Part model, mm, in its own coordinate system. Face numbers are marked on the shaded views. A direction names the side the tool comes from. Give positions to 0.01 mm unless a question says otherwise; leave off trailing zeros. Write each loop counter-clockwise with the first axis right and the second up, starting at its lowest first coordinate (ties: lowest second). Pieces come first, ordered by that corner, then holes.
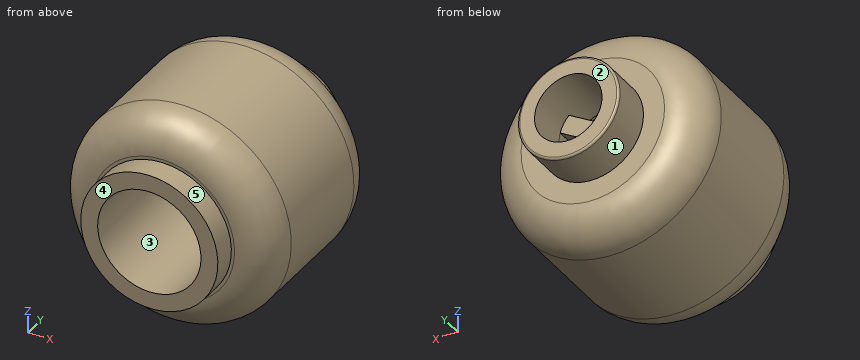
```python
from build123d import *

# Parameters (mm, degrees)
FILLET1_R          = 1.7
SKETCH2_R          = 1.6
CUT_EXTRUDE1_DEPTH = 2
CUT_EXTRUDE2_DEPTH = 13.0074977
SKETCH4_R          = 2.45
CUT_EXTRUDE3_DEPTH = 8.5
FILLET2_R          = 0.1


with BuildPart() as part:
    # Sketch1 → Revolve1 (revolve)
    with BuildSketch(Plane.XY, mode=Mode.PRIVATE) as revolve1_sk:
        Polygon((0, 11.6), (2.4, 11.6), (2.4, 9.6), (5.1, 9.6), (5.1, 1.1), (3.25, 1.1), (3.25, 0), (0, 0), align=None)
    revolve(revolve1_sk.sketch.rotate(Axis((0, 161.315789474, 0), (0, -1, 0)), 90), axis=Axis((0, 161.315789474, 0), (0, -1, 0)))

    # Fillet1
    fillet1_edges = [part.edges().sort_by_distance(p)[0] for p in [
        (0, 1.1, -5.1),
        (0, 9.6, -5.1),
    ]]
    fillet(fillet1_edges, radius=FILLET1_R)

    # Sketch2 → Cut-Extrude1 (cut)
    with BuildSketch(Plane(origin=(0, 11.6, 0), x_dir=(1, 0, 0), z_dir=(0, 1, 0))):
        with Locations(Location((0, 0, 0), (0, 0, 270))):
            Circle(SKETCH2_R)
    extrude(amount=-CUT_EXTRUDE1_DEPTH, mode=Mode.SUBTRACT)

    # Sketch3 → Cut-Extrude2 (cut, through all)
    with BuildSketch(Plane(origin=(0, 9.6, 0), x_dir=(1, 0, 0), z_dir=(0, 1, 0))):
        with BuildLine():
            Line((-0.42, 0.242487113), (-0.42, 1.543891188))
            ThreePointArc((-0.42, 1.543891188), (-1.385640646, 0.8), (-1.547048989, -0.408214924))
            Line((-1.547048989, -0.408214924), (-0.42, 0.242487113))
        make_face()
        with BuildLine():
            ThreePointArc((1.6, 0), (1.271219887, 0.971596624), (0.42, 1.543891188))
            Line((0.42, 1.543891188), (0.42, 0.242487113))
            Line((0.42, 0.242487113), (1.547048989, -0.408214924))
            ThreePointArc((1.547048989, -0.408214924), (1.586707028, -0.205817415), (1.6, 0))
        make_face()
        with BuildLine():
            Line((0, -0.484974226), (-1.127048989, -1.135676264))
            ThreePointArc((-1.127048989, -1.135676264), (0, -1.6), (1.127048989, -1.135676264))
            Line((1.127048989, -1.135676264), (0, -0.484974226))
        make_face()
    extrude(amount=-CUT_EXTRUDE2_DEPTH, mode=Mode.SUBTRACT)

    # Sketch4 → Cut-Extrude3 (cut)
    with BuildSketch(Plane.XZ):
        with Locations(Location((0, 0, 0), (0, 0, 270))):
            Circle(SKETCH4_R)
    extrude(amount=-CUT_EXTRUDE3_DEPTH, mode=Mode.SUBTRACT)

    # Fillet2
    fillet2_edges = [part.edges().sort_by_distance(p)[0] for p in [
        (0, 11.6, -2.4),
    ]]
    fillet(fillet2_edges, radius=FILLET2_R)


solid = part.part
```
1) Saw through at B-B, the plane x = 0.75. Count the separate pieces of the cut face and the enclosed holes in it, then the cut area to 3 significant figures.
Answers follow:
separate pieces: 3
enclosed holes: 0
area: 52.0 mm2
2) 3-axis set-ups, long thin cutter, end or side, ignore diameter. For the marked faces 1 and 2: which of +Z, -Z, +X, -X, +Y, -Y reach the whole face in a straight line?
Answers follow:
face 1: +Y
face 2: +Z, -Z, +X, -X, +Y
3) Pin check, flat tips, straight feed: pin 1 Ø0.9 at (y, z) = (9, -1) entering from -X; pin 2 Ø3 at (x, z) = (0, 0) entering from -Y; pin 3 Ø2 at (y, z) = (9, 1) entering from +X. Stop position of each tip, or through.
Answers follow:
pin 1: stops at x = -4.89
pin 2: stops at y = 8.5
pin 3: stops at x = 5.06
4) Saw through at D-D, the plane y = 2.5. Write the cut outline in (x, z).
Answers follow:
outline: circle Ø10.15 at (0, 0); hole circle Ø4.9 at (0, 0)
5) Wall check: L1, parallel to X at y = 6, z = 0; L2, parallel to Z at x = -2, y = 7.75; L3, parallel to Y at x = -1.75, z = 0.75. Give the ranges that are in metal, low to high.
Answers follow:
L1: x = -5.1 to -2.45, 2.45 to 5.1
L2: z = -4.69 to -1.42, 1.42 to 4.69
L3: y = 8.5 to 11.6
6) Two-plate mould, pull along X, no slides. Class the marked faces 3, 4 and 5: +X half, -X half, draft (parallel to the pull), parting line (faces both ways), or undercut.
Answers follow:
face 3: undercut
face 4: draft
face 5: parting line
7) Saw through at A-A, the plane y = 9.75. Write the cut outline in (x, z), then the cut area to 3 significant figures.
Answers follow:
outline: circle Ø4.8 at (0, 0); hole circle Ø3.2 at (0, 0)
area: 10.1 mm2
